Check sheet for the drawn part. Datum: minimum x, y, z corner. Units: mm. A direction names the side the tool comes from. Round coordinates to 2 decimals unless told otherwise and drop trailing zeros. Write each loop counter-clockwise with the first axis right and the second up, starting at its lowest first coordinate (ties: lowest second). Pieces come first, ordered by that corner, then holes. Notation, with made-up numbers: (-11, 4) - (15, 4) arc R20 ccw to (15, 17) - close; hole circle Ø5 at (45.25, -28). An arc over 180 degrees is marked (long way). Write each question's results on one line, items separated by ' | '.
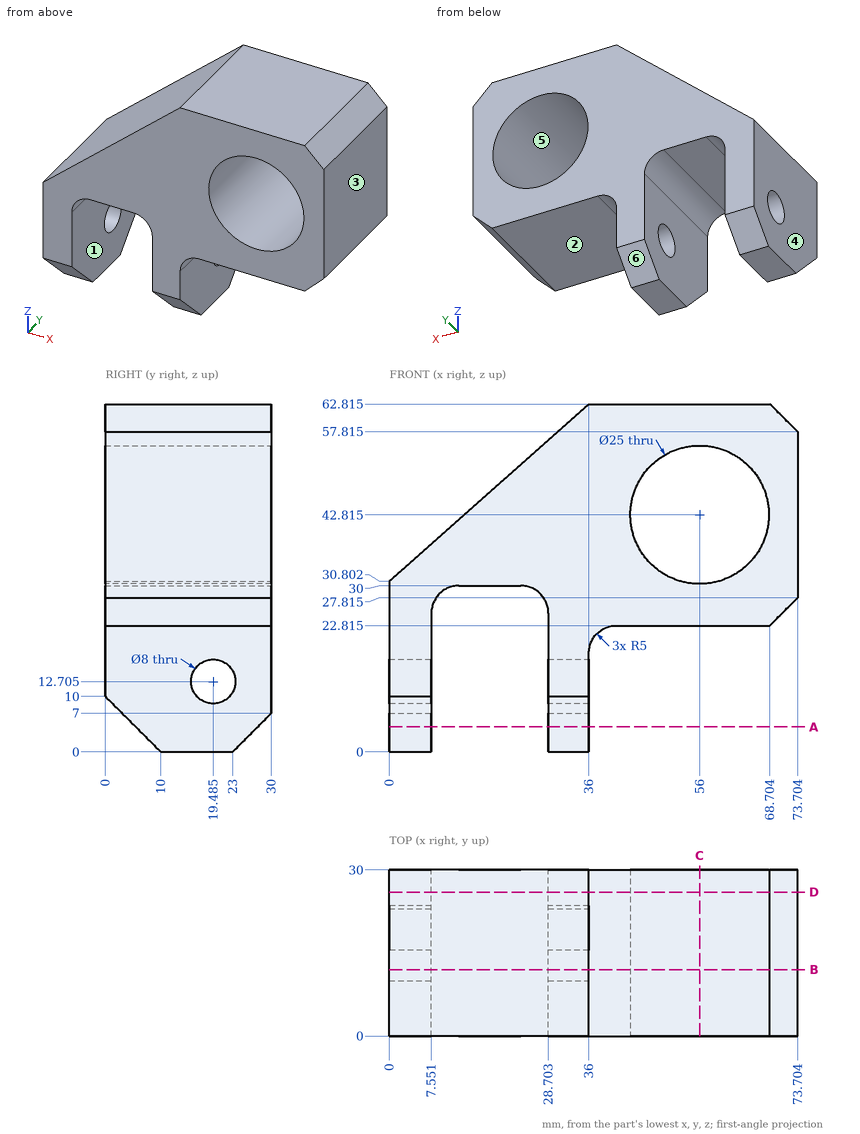
(1) Section check C-C (x = 56). Record the cut outline in (y, z) (1 decimal), plus the area to 3 significant figures.
Answer:
outline: (0, 22.8) - (30, 22.8) - (30, 30.3) - (0, 30.3) - close; (0, 55.3) - (30, 55.3) - (30, 62.8) - (0, 62.8) - close | area: 450 mm2
(2) Section check B-B (y = 12). Record the cut outline in (x, z) (1 decimal), plus the area to 3 significant figures.
Answer:
outline: (0, 0) - (7.6, 0) - (7.6, 25) arc R5 cw to (12.6, 30) - (23.7, 30) arc R5 cw to (28.7, 25) - (28.7, 0) - (36, 0) - (36, 17.8) arc R5 cw to (41, 22.8) - (68.7, 22.8) - (73.7, 27.8) - (73.7, 57.8) - (68.7, 62.8) - (36, 62.8) - (0, 30.8) - close; hole circle Ø25 at (56, 42.8) | area: 2,060 mm2
(3) Thickness scan on L1, parallel to Y at x = 4.5, z = 13 (1 decimal); L2, parallel to X at y = 25, z = 12.5; L3, parallel to Z at x = 65, y = 21.5 (1 decimal). Record the ranges inside material, lowest first.
Answer:
L1: 0 to 15.5, 23.5 to 30 | L2: 0 to 7.55, 28.7 to 36 | L3: 22.8 to 34.1, 51.5 to 62.8
(4) Go/stop test with flat-tipped pins: pin 1 Ø13 at (y, z) = (19.48, 12.71) entering from -X; pin 2 Ø8 at (x, y) = (54, 6) entering from -Z (1 decimal); pin 3 Ø9 at (x, y) = (18.5, 8.5) entering from -Z; pin 4 Ø6 at (x, y) = (11.5, 4.5) entering from +Z (1 decimal). Record where each tip stops, or that it passes through.
Answer:
pin 1: x = 0 | pin 2: z = 22.8 | pin 3: z = 30 | pin 4: z = 43.7
(5) Set-up check for the marked faces 1, 2 and 3: record each of +Z, -Z, +X, -X, +Y, -Y from which the full face is reachable in a straight line by a thin tool's end or side.
Answer:
face 1: -Z, +Y, -Y | face 2: -Z, +X, +Y, -Y | face 3: +Z, -Z, +X, +Y, -Y
(6) Section check D-D (y = 26). Record the cut outline in (x, z) (1 decimal), plus the area to 3 significant figures.
Answer:
outline: (0, 3) - (7.6, 3) - (7.6, 25) arc R5 cw to (12.6, 30) - (23.7, 30) arc R5 cw to (28.7, 25) - (28.7, 3) - (36, 3) - (36, 17.8) arc R5 cw to (41, 22.8) - (68.7, 22.8) - (73.7, 27.8) - (73.7, 57.8) - (68.7, 62.8) - (36, 62.8) - (0, 30.8) - close; hole circle Ø25 at (56, 42.8) | area: 2,010 mm2
(7) Mould release check, pull along Z, two halves, no side actions. Record for the marked faces 4, 5 and 6: released by +Z, released by -Z, zero draft, split by the parting line, or undercut.
Answer:
face 4: zero draft | face 5: undercut | face 6: released by -Z
(8) Section check A-A (z = 4.5). Record the cut outline in (x, y).
Answer:
outline: (0, 5.5) - (7.55, 5.5) - (7.55, 27.5) - (0, 27.5) - close; (28.7, 5.5) - (36, 5.5) - (36, 27.5) - (28.7, 27.5) - close
